Can you work these out from the model? Positions are in its coordinate system, mm. A direction names the side the tool comes from. Coordinates: 2 decimals unless noted, no trailing zeros. Loops run counter-clockwise (first coordinate to the right, second up) from the corner with the lowest first, then second, coordinate; pieces in that order, holes last.
```python
from build123d import *

# Parameters (mm, degrees)
ESBO_O1_W                = 23
ESBO_O1_H                = 12
RESSALTO_EXTRUS_O1_DEPTH = 26
ESBO_O8_W                = 23
ESBO_O8_H                = 12
ESBO_O8_W_2              = 22.98
ESBO_O8_H_2              = 11.98
CORTE_EXTRUS_O3_DEPTH    = 10
ESBO_O2_R                = 4.239559465
RESSALTO_EXTRUS_O2_DEPTH = 1
ESBO_O3_R                = 2.5
CORTE_EXTRUS_O1_DEPTH    = 1
ESBO_O4_R                = 2.4
RESSALTO_EXTRUS_O3_DEPTH = 5
ESBO_O5_W                = 12
ESBO_O5_H                = 1
RESSALTO_EXTRUS_O4_DEPTH = 4.5
ESBO_O6_R                = 1.4
CORTE_EXTRUS_O2_DEPTH    = 4.5
FILETE1_R                = 0.5
FILETE2_R                = 0.2
FILETE1_OF_ESPELHAR1_R   = 0.5
FILETE2_OF_ESPELHAR1_R   = 0.2
FILETE3_R                = 0.8
CHANFRO1_SIZE            = 1
FILETE4_R                = 0.4
FILETE5_R                = 0.4
FILETE6_R                = 0.4


with BuildPart() as part:
    # Esboço1 → Ressalto-extrusão1 (new body)
    with BuildSketch(Plane(origin=(0, 0, 0), x_dir=(1, 0, 0), z_dir=(0, 1, 0))):
        Rectangle(ESBO_O1_W, ESBO_O1_H)
    extrude(amount=RESSALTO_EXTRUS_O1_DEPTH)

    # Esboço8 → Corte-extrusão3 (cut)
    with BuildSketch(Plane(origin=(0, 8, 0), x_dir=(-1, 0, 0), z_dir=(0, -1, 0))):
        Rectangle(ESBO_O8_W, ESBO_O8_H)
        Rectangle(ESBO_O8_W_2, ESBO_O8_H_2, mode=Mode.SUBTRACT)
    extrude(amount=-CORTE_EXTRUS_O3_DEPTH, mode=Mode.SUBTRACT)

    # Esboço2 → Ressalto-extrusão2 (add)
    with BuildSketch(Plane(origin=(0, 26, 0), x_dir=(1, 0, 0), z_dir=(0, 1, 0))):
        with Locations(Location((-5.5, 0, 0), (0, 0, 90))):
            Circle(ESBO_O2_R)
    extrude(amount=RESSALTO_EXTRUS_O2_DEPTH)

    # Esboço3 → Corte-extrusão1 (cut)
    with BuildSketch(Plane(origin=(0, 27, 0), x_dir=(1, 0, 0), z_dir=(0, 1, 0))):
        with Locations(Location((-5.5, 0, 0), (0, 0, 270))):
            Circle(ESBO_O3_R)
    extrude(amount=-CORTE_EXTRUS_O1_DEPTH, mode=Mode.SUBTRACT)

    # Esboço4 → Ressalto-extrusão3 (add)
    with BuildSketch(Plane(origin=(0, 26, 0), x_dir=(1, 0, 0), z_dir=(0, 1, 0))):
        with Locations(Location((-5.5, 0, 0), (0, 0, 270))):
            Circle(ESBO_O4_R)
    extrude(amount=RESSALTO_EXTRUS_O3_DEPTH)

    # Esboço5 → Ressalto-extrusão4 (add)
    with BuildSketch(Plane(origin=(11.5, 0, 0), x_dir=(0, 0, -1), z_dir=(1, 0, 0))):
        with Locations((0, 20.5)):
            Rectangle(ESBO_O5_W, ESBO_O5_H)
    ressalto_extrus_o4 = extrude(amount=RESSALTO_EXTRUS_O4_DEPTH)

    # Esboço6 → Corte-extrusão2 (cut)
    with BuildSketch(Plane(origin=(0, 21, 0), x_dir=(1, 0, 0), z_dir=(0, 1, 0))):
        with Locations(Location((13.75, 3.5, 0), (0, 0, 270))):
            Circle(ESBO_O6_R)
        with Locations(Location((13.75, -3.5, 0), (0, 0, 270))):
            Circle(ESBO_O6_R)
        with BuildLine():
            Line((13.75, 1), (16, 1))
            Line((16, 1), (16, -1))
            Line((16, -1), (13.75, -1))
            ThreePointArc((13.75, -1), (12.75, 0), (13.75, 1))
        make_face()
    corte_extrus_o2 = extrude(amount=-CORTE_EXTRUS_O2_DEPTH, mode=Mode.SUBTRACT)

    # Filete1
    filete1_edges = [part.edges().sort_by_distance(p)[0] for p in [
        (16, 20.5, -6),
        (16, 20.5, 6),
    ]]
    fillet(filete1_edges, radius=FILETE1_R)

    # Filete2
    filete2_edges = [part.edges().sort_by_distance(p)[0] for p in [
        (16, 20.5, 1),
        (16, 20.5, -1),
    ]]
    fillet(filete2_edges, radius=FILETE2_R)

    # Espelhar1: Ressalto-extrusão4, Corte-extrusão2 across plane
    add(ressalto_extrus_o4.mirror(Plane(origin=(0, 0, 0), x_dir=(0, 0, 1), z_dir=(1, 0, 0))))
    add(corte_extrus_o2.mirror(Plane(origin=(0, 0, 0), x_dir=(0, 0, 1), z_dir=(1, 0, 0))), mode=Mode.SUBTRACT)

    # Filete1 of Espelhar1
    filete1_of_espelhar1_edges = [part.edges().sort_by_distance(p)[0] for p in [
        (-16, 20.5, -6),
        (-16, 20.5, 6),
    ]]
    fillet(filete1_of_espelhar1_edges, radius=FILETE1_OF_ESPELHAR1_R)

    # Filete2 of Espelhar1
    filete2_of_espelhar1_edges = [part.edges().sort_by_distance(p)[0] for p in [
        (-16, 20.5, 1),
        (-16, 20.5, -1),
    ]]
    fillet(filete2_of_espelhar1_edges, radius=FILETE2_OF_ESPELHAR1_R)

    # Filete3
    filete3_edges = [part.edges().sort_by_distance(p)[0] for p in [
        (-11.5, 23.5, -6),
        (-11.5, 4, -6),
        (-11.5, 19, -6),
        (11.5, 4, -6),
        (11.5, 19, -6),
        (11.5, 23.5, -6),
        (-11.5, 4, 6),
        (-11.5, 19, 6),
        (-11.5, 23.5, 6),
        (11.5, 23.5, 6),
        (11.5, 4, 6),
        (11.5, 19, 6),
        (-11.49, 13, 5.99),
        (-11.49, 13, -5.99),
        (11.49, 13, -5.99),
        (11.49, 13, 5.99),
    ]]
    fillet(filete3_edges, radius=FILETE3_R)

    # Chanfro1
    # the kernel refuses this chamfer: 1 mm, written as the material it takes off along each edge
    with BuildSketch(Plane(origin=(11.5, 26, 7.771682988), x_dir=(-0.9996219169112968, 0.027495876610585647, 0), z_dir=(0, 0, -1))) as chanfro1_piece_1:
        Polygon((CHANFRO1_SIZE * 0.999621916911, -CHANFRO1_SIZE * 0.0274958766106), (-CHANFRO1_SIZE * 0.0274958766106, -CHANFRO1_SIZE * 0.999621916911), (0, 0), align=None)
    extrude(amount=15.543365976, mode=Mode.SUBTRACT)

    # Filete4
    # the kernel refuses this fillet: 0.4 mm, written as the material it takes off along each edge
    with BuildSketch(Plane(origin=(11.5, 26, -6), x_dir=(0, -1, 0), z_dir=(-1, 0, 0)), Plane(origin=(-10.7, 26, 6), x_dir=(0, -1, 0), z_dir=(1, 0, 0))) as filete4_piece_1:
        with BuildLine():
            CenterArc((FILETE4_R, FILETE4_R), FILETE4_R, 180, 90)
            Line((0, FILETE4_R), (0, 0))
            Line((0, 0), (FILETE4_R, 0))
        make_face()
    extrude(amount=22.2, mode=Mode.SUBTRACT)
    with BuildSketch(Plane(origin=(-10.7, 26, -5.2), x_dir=(0, 0, -1), z_dir=(1, 0, 0))) as filete4_piece_2:
        with BuildLine():
            CenterArc((0.8 - FILETE4_R, -FILETE4_R), FILETE4_R, 0, 90)
            Line((0.8 - FILETE4_R, 0), (0.8, 0))
            Line((0.8, 0), (0.8, -FILETE4_R))
        make_face()
    revolve(axis=Axis((-10.7, 26, -5.2), (0, 1, 0)), revolution_arc=90, mode=Mode.SUBTRACT)
    with BuildSketch(Plane(origin=(-11.5, 26, -5.2), x_dir=(1, 0, 0), z_dir=(0, 0, 1)), Plane(origin=(-11.5, 0, -5.2), x_dir=(0, 1, 0), z_dir=(0, 0, 1)), Plane(origin=(11.5, 0, 5.2), x_dir=(0, 1, 0), z_dir=(0, 0, -1))) as filete4_piece_3:
        with BuildLine():
            CenterArc((FILETE4_R, -FILETE4_R), FILETE4_R, 90, 90)
            Line((0, -FILETE4_R), (0, 0))
            Line((0, 0), (FILETE4_R, 0))
        make_face()
    extrude(amount=10.4, mode=Mode.SUBTRACT)
    with BuildSketch(Plane(origin=(-10.7, 26, 5.2), x_dir=(0, 0, 1), z_dir=(1, 0, 0))) as filete4_piece_4:
        with BuildLine():
            CenterArc((0.8 - FILETE4_R, FILETE4_R), FILETE4_R, 270, 90)
            Line((0.8, FILETE4_R), (0.8, 0))
            Line((0.8, 0), (0.8 - FILETE4_R, 0))
        make_face()
    revolve(axis=Axis((-10.7, 26, 5.2), (0, -1, 0)), revolution_arc=90, mode=Mode.SUBTRACT)
    with BuildSketch(Plane(origin=(10.7, 0, -6), x_dir=(0, 1, 0), z_dir=(-1, 0, 0)), Plane(origin=(-10.7, 0, 6), x_dir=(0, 1, 0), z_dir=(1, 0, 0))) as filete4_piece_5:
        with BuildLine():
            CenterArc((FILETE4_R, -FILETE4_R), FILETE4_R, 90, 90)
            Line((0, -FILETE4_R), (0, 0))
            Line((0, 0), (FILETE4_R, 0))
        make_face()
    extrude(amount=21.4, mode=Mode.SUBTRACT)
    with BuildSketch(Plane(origin=(-10.7, 0, 5.2), x_dir=(0, 0, 1), z_dir=(1, 0, 0))) as filete4_piece_6:
        with BuildLine():
            CenterArc((0.8 - FILETE4_R, -FILETE4_R), FILETE4_R, 0, 90)
            Line((0.8 - FILETE4_R, 0), (0.8, 0))
            Line((0.8, 0), (0.8, -FILETE4_R))
        make_face()
    revolve(axis=Axis((-10.7, 0, 5.2), (0, -1, 0)), revolution_arc=90, mode=Mode.SUBTRACT)
    with BuildSketch(Plane(origin=(-10.7, 0, -5.2), x_dir=(0, 0, -1), z_dir=(1, 0, 0))) as filete4_piece_7:
        with BuildLine():
            CenterArc((0.8 - FILETE4_R, FILETE4_R), FILETE4_R, 270, 90)
            Line((0.8 - FILETE4_R, 0), (0.8, 0))
            Line((0.8, 0), (0.8, FILETE4_R))
        make_face()
    revolve(axis=Axis((-10.7, 0, -5.2), (0, 1, 0)), revolution_arc=90, mode=Mode.SUBTRACT)
    with BuildSketch(Plane(origin=(10.7, 0, -5.2), x_dir=(0, 0, -1), z_dir=(-1, 0, 0))) as filete4_piece_8:
        with BuildLine():
            CenterArc((0.8 - FILETE4_R, -FILETE4_R), FILETE4_R, 0, 90)
            Line((0.8 - FILETE4_R, 0), (0.8, 0))
            Line((0.8, 0), (0.8, -FILETE4_R))
        make_face()
    revolve(axis=Axis((10.7, 0, -5.2), (0, -1, 0)), revolution_arc=90, mode=Mode.SUBTRACT)
    with BuildSketch(Plane(origin=(10.7, 0, 5.2), x_dir=(1, 0, 0), z_dir=(0, 0, -1))) as filete4_piece_9:
        with BuildLine():
            CenterArc((0.8 - FILETE4_R, -FILETE4_R), FILETE4_R, 0, 90)
            Line((0.8 - FILETE4_R, 0), (0.8, 0))
            Line((0.8, 0), (0.8, -FILETE4_R))
        make_face()
    revolve(axis=Axis((10.7, 0, 5.2), (0, -1, 0)), revolution_arc=90, mode=Mode.SUBTRACT)

    # Filete5
    filete5_edges = [part.edges().sort_by_distance(p)[0] for p in [
        (-5.5, 27, 4.239559465),
    ]]
    fillet(filete5_edges, radius=FILETE5_R)

    # Filete6
    filete6_edges = [part.edges().sort_by_distance(p)[0] for p in [
        (-5.5, 26, 4.239559465),
    ]]
    fillet(filete6_edges, radius=FILETE6_R)


solid = part.part
```
Item 1: We'd pull the mould along X, two halves only. Please class faces 1 (the face through (-11.5, 4, 0)), 2 (the face through (14.9, 20.5, -2.7)), 3 (the face through (14.9, 20.5, 4.3)), 4 (the face through (0, 22, -6)): +X half, -X half, draft (parallel to the pull), parting line (faces both ways), or undercut.
Results are:
face 1: -X half
face 2: undercut
face 3: undercut
face 4: draft
Item 2: On a 3-axis mill with a long thin cutter (end or side, diameter ignored), from which of +Z, -Z, +X, -X, +Y, -Y can I reach the whole of each face in a straight line? I mean faces 5 (the face through (11.27, 4.25, -5.76)), 6 (the face through (14.8, 20.5, 1)), 7 (the face through (-11.26, 23.33, 5.77)), 8 (the face through (-6, 27, -3)). Say none if no direction works.
Results are:
face 5: -Z, +X, -Y
face 6: +X, +Y, -Y
face 7: +Z, -X, +Y
face 8: +Y
Item 3: Suppose I cut it at D-D, the plane y = 12. Please give me the cut outline in (x, z).
Results are:
outline: (-11.49, -5.19) arc R0.8 ccw to (-10.69, -5.99) - (10.69, -5.99) arc R0.8 ccw to (11.49, -5.19) - (11.49, 5.19) arc R0.8 ccw to (10.69, 5.99) - (-10.69, 5.99) arc R0.8 ccw to (-11.49, 5.19) - close
Item 4: I need wall thicknesses on line 1 along X through (y, z) = (20.5, 3.5); line 2 along Z through (x, y) = (-13.75, 20.3); line 3 along X through (y, z) = (6, 0). Which ranges of each line are inside material? Lowest first, please.
Results are:
line 1: x = -16 to -15.15, -12.35 to 12.35, 15.15 to 16
line 2: z = -6 to -4.9, -2.1 to -1, 1 to 2.1, 4.9 to 6
line 3: x = -11.5 to 11.5
Item 5: I'm going to push flat-ended pins straight in: P1, Ø4, axis at x = -13, z = 2.5, coming from the +Y side; P2, Ø1, axis at y = 19, z = -1, coming from the +X side; P3, Ø3.5, axis at x = -13.75, z = -3.5, coming from the +Y side; P4, Ø1.7, axis at x = -13.75, z = 3.5, coming from the -Y side (3 decimals). Where does each tip first touch, or does it pass through?
Results are:
P1: stops at y = 26
P2: stops at x = 11.5
P3: stops at y = 21
P4: passes through
Item 6: Suppose I cut it at B-B, the plane y = 19.5. Please give me the cut outline in (x, z), plus the area to 3 significant figures.
Results are:
outline: (-11.5, -5.2) arc R0.8 ccw to (-10.7, -6) - (10.7, -6) arc R0.8 ccw to (11.5, -5.2) - (11.5, 5.2) arc R0.8 ccw to (10.7, 6) - (-10.7, 6) arc R0.8 ccw to (-11.5, 5.2) - close
area: 275 mm2
